Check sheet for the drawn part. Datum: minimum x, y, z corner. Units: mm. Give positions to 0.01 mm unless a question says otherwise; leave off trailing zeros. Loops run counter-clockwise (first coordinate to the right, second up) from the corner with the lowest first, then second, coordinate; pieces in that order, holes last. Notation, with made-up numbers: (72, 73.25) - (94, 73.25) arc R30 cw to (94, 106.25) - close; hole circle Ø7 at (84, -27). An arc over 180 degrees is marked (long way). One line per item, written item: value. Start each with the question number.
1. Gauge pin test, flat ends, axial feed: pin 1 (1.5 mm diameter, centred on y = 1, z = 15.5, fed in from -X); pin 2 (3 mm diameter, centred on x = 4, y = 4, fed in from -Z); pin 3 (1.5 mm diameter, centred on x = 7, z = 11, fed in from +Y). Record the tip position at first contact, or that the pin passes through.
2. Sectioned sample at D-D (z = 14). Record the cut outline in (x, y), plus the area to 3 significant figures.
3. Mould release check, pull along Y, two halves, no side actions. Record for the marked faces 1, 2 and 3: pulls with the +Y half, pulls with the -Y half, needs draft (parallel to the pull), parting line crosses it, or undercut.
4. Sectioned sample at A-A (y = 4). Record the cut outline in (x, z), plus the area to 4 significant figures.
5. Scan lines: L1, parallel to Y at x = 4, z = 7.6; L2, parallel to Y at x = 4, z = 3.1; L3, parallel to X at y = 5.5, z = 8.75. Record each from-to range of solid material in increasing order. Write a range as [from, to].
6. Sectioned sample at B-B (z = 5.75). Record the cut outline in (x, y), plus the area to 3 significant figures.
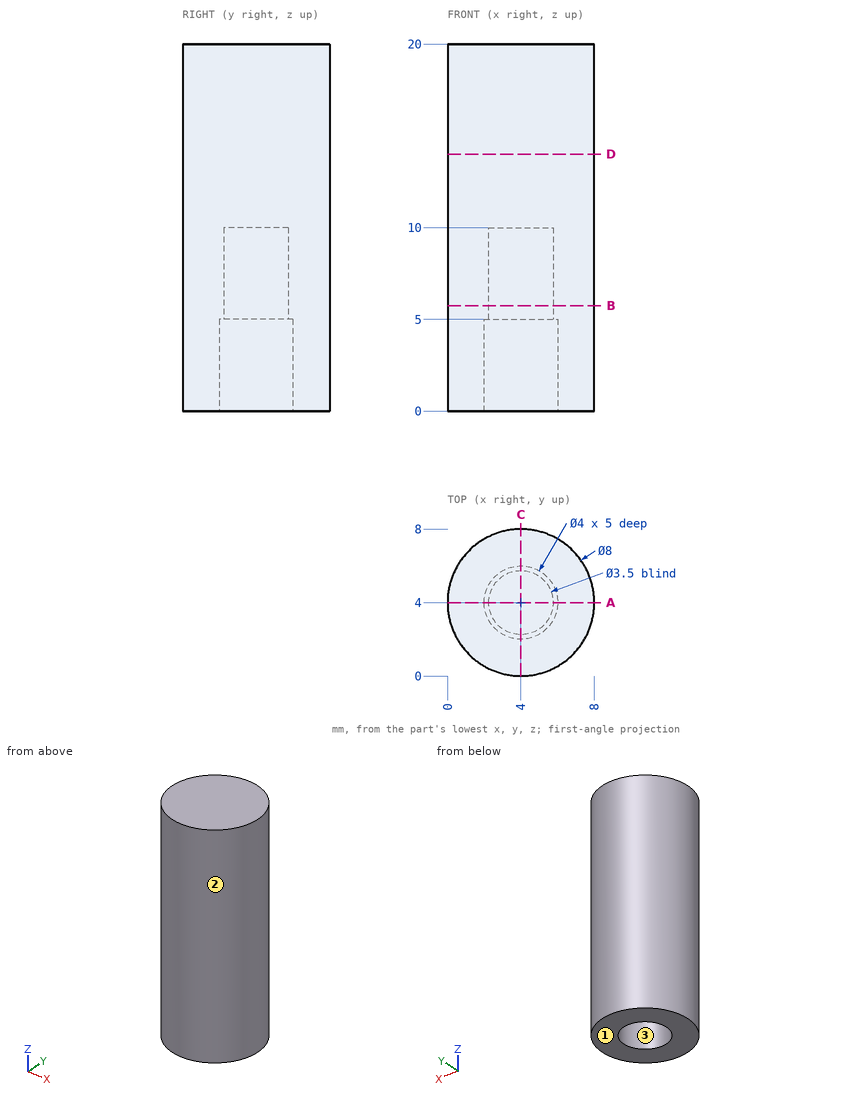
Results are:
1. pin 1: stops at x = 0.69
1. pin 2: stops at z = 10
1. pin 3: stops at y = 7.31
2. outline: circle Ø8 at (4, 4)
2. area: 50.3 mm^2
3. face 1: needs draft
3. face 2: parting line crosses it
3. face 3: undercut
4. outline: (0, 0) - (2, 0) - (2, 5) - (2.25, 5) - (2.25, 10) - (5.75, 10) - (5.75, 5) - (6, 5) - (6, 0) - (8, 0) - (8, 20) - (0, 20) - close
4. area: 122.5 mm^2
5. L1: y = [0, 2.25], [5.75, 8]
5. L2: y = [0, 2], [6, 8]
5. L3: x = [0.29, 3.1], [4.9, 7.71]
6. outline: circle Ø8 at (4, 4); hole circle Ø3.5 at (4, 4)
6. area: 40.6 mm^2
